Here's the drawing with two shaded views (mm, measured from the low corner). I have some questions. A direction names the side the tool comes from. Give positions to 0.01 mm unless a question says otherwise; leave off trailing zeros. Loops run counter-clockwise (first coordinate to the right, second up) from the corner with the lowest first, then second, coordinate; pieces in that order, holes last. Notation, with made-up numbers: (-35, 56) -> (24, 56) arc R21 cw to (24, 91) -> close; hole circle Ø10 at (23, 26). An arc over 180 degrees is marked (long way). Answer in a Markdown table with one row per item. Add a question column.
Item 1: If we section it at A-A (x = 43): Write out the boundary of the cut face in (y, z).
Item 2: If I drill on line 1 (X direction, y = 18.5, z = 6.25); line 2 (Y direction, x = 52, z = 8.25); line 3 (X direction, y = 36.5, z = 23), over which ranges is the centre line in solid material (lowest first)?
Item 3: We'd pull the mould along X, two halves only. Please class the marked faces 3, 4, 5 and 6: released by +X, released by -X, zero draft, split by the parting line, or undercut.
Item 4: Which directions (+Z, -Z, +X, -X, +Y, -Y) give clear straight access to the entire face, cutting with the end or side of a thin tool? Please do the marked faces 1 and 2.
Item 5: If we section it at D-D (x = 19.5): Write out the boundary of the cut face in (y, z), then the cut area to 3 significant figures.
Item 6: If we section it at C-C (y = 14): Write out the boundary of the cut face in (x, z).
Item 7: For P1, Ø10, axis at y = 22.5, z = 23, coming from the +X side; P2, Ø8, axis at y = 21.5, z = 19, coming from the -X side; P3, Ø4.5, axis at x = 37.5, y = 36.5, coming from the +Z side; P4, Ø3, axis at x = 36, y = 35.5, coming from the -Z side, each with a flat end and sliding along its axis, tell me the tip position at first contact or that it passes through.
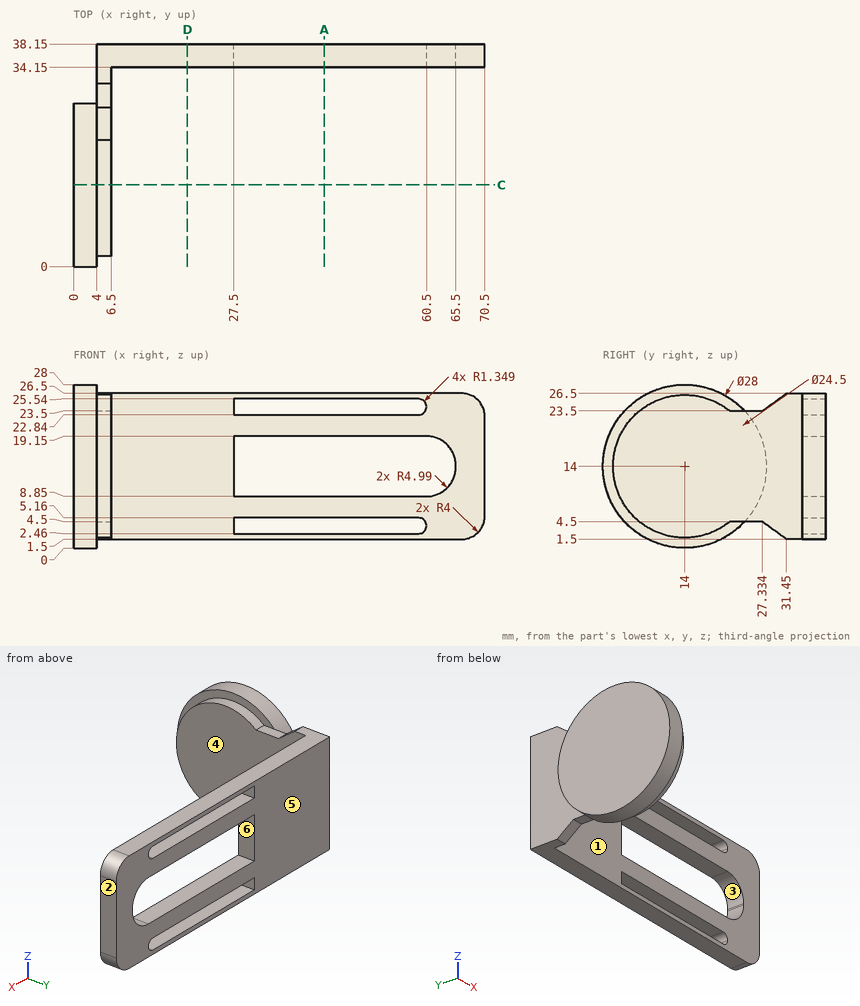
Recorded:
| question | item | result |
|---|---|---|
| 1 | outline | (34.15, 1.5) -> (38.15, 1.5) -> (38.15, 2.46) -> (34.15, 2.46) -> close; (34.15, 5.16) -> (38.15, 5.16) -> (38.15, 8.85) -> (34.15, 8.85) -> close; (34.15, 19.15) -> (38.15, 19.15) -> (38.15, 22.84) -> (34.15, 22.84) -> close; (34.15, 25.54) -> (38.15, 25.54) -> (38.15, 26.5) -> (34.15, 26.5) -> close |
| 2 | line 1 | x = 0 to 6.5 |
| 2 | line 2 | y = 34.15 to 38.15 |
| 2 | line 3 | x = 4 to 27.5, 59.79 to 70.47 |
| 3 | face 3 | undercut |
| 3 | face 4 | released by +X |
| 3 | face 5 | zero draft |
| 3 | face 6 | undercut |
| 4 | face 1 | +Z, -Z, +X, -Y |
| 4 | face 2 | +Z, -Z, +X, +Y, -Y |
| 5 | outline | (34.15, 1.5) -> (38.15, 1.5) -> (38.15, 26.5) -> (34.15, 26.5) -> close |
| 5 | area | 100 mm^2 |
| 6 | outline | (0, 0) -> (4, 0) -> (4, 1.75) -> (6.5, 1.75) -> (6.5, 26.25) -> (4, 26.25) -> (4, 28) -> (0, 28) -> close |
| 7 | P1 | stops at x = 6.5 |
| 7 | P2 | stops at x = 0 |
| 7 | P3 | stops at z = 26.5 |
| 7 | P4 | stops at z = 1.5 |
